Geometry: final body of the model. Coordinates: model frame, mm. Face numbers are marked on the shaded views. A direction names the side the tool comes from. Give positions to 0.01 mm unless a question says otherwise; leave off trailing zeros. Write each loop counter-clockwise with the first axis right and the second up, starting at its lowest first coordinate (ties: lowest second). Pieces come first, ordered by that corner, then holes. Notation, with made-up numbers: (4, 59.25) - (25, 59.25) arc R18 cw to (25, 86.25) - close; hole circle Ø11 at (-19, 79). An arc over 180 degrees is marked (long way). One line per question, with ' | ' between items. Start each with the question number.
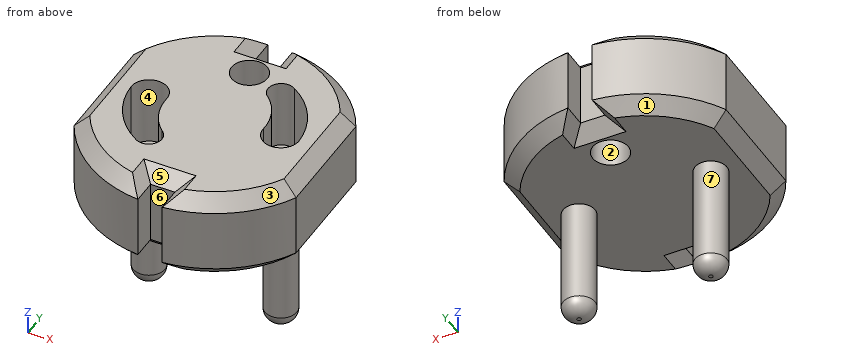
```python
from build123d import *

# Parameters (mm, degrees)
F0_R     = 2.575
F1_DEPTH = 13
F0_R_2   = 2.3
F2_DEPTH = 3
F3_DEPTH = 17
F4_R     = 2
F5_SIZE  = 1.99999
F6_SIZE  = 1.99999


# Not quite as in the source:
# - a fillet or chamfer is up to 0.001 mm smaller than in the source, because OpenCascade refuses the exact size


with BuildPart() as f1:
    # F0 (on Top) → F1 (new body)
    with BuildSketch(Plane.XY):
        with BuildLine():
            Line((1.75, -14.4147285773), (1.75, -17.9147285773))
            ThreePointArc((1.75, -17.9147285773), (10.1062199571, -14.895110546), (16, -8.2462112512))
            Line((16, -8.2462112512), (16, 8.2462112512))
            ThreePointArc((16, 8.2462112512), (10.1062199571, 14.895110546), (1.75, 17.9147285773))
            Line((1.75, 17.9147285773), (1.75, 14.4147285773))
            Line((1.75, 14.4147285773), (-1.75, 14.4147285773))
            Line((-1.75, 14.4147285773), (-1.75, 17.9147285773))
            ThreePointArc((-1.75, 17.9147285773), (-10.1062199571, 14.895110546), (-16, 8.2462112512))
            Line((-16, 8.2462112512), (-16, -8.2462112512))
            ThreePointArc((-16, -8.2462112512), (-10.1062199571, -14.895110546), (-1.75, -17.9147285773))
            Line((-1.75, -17.9147285773), (-1.75, -14.4147285773))
            Line((-1.75, -14.4147285773), (1.75, -14.4147285773))
        make_face()
        with BuildLine():
            ThreePointArc((-12.1, 0), (-9.4098118123, 2.5984353159), (-6.9062568532, -0.1802678246))
            ThreePointArc((-6.9062568532, -0.1802678246), (-6.3236870302, -3.4718300474), (-4.3937995375, -6.2011713107))
            ThreePointArc((-4.3937995375, -6.2011713107), (-3.9419565942, -8.8499140227), (-6.5906993063, -9.301756966))
            ThreePointArc((-6.5906993063, -9.301756966), (-10.5283348632, -5.3515440951), (-12.1, 0))
        make_face(mode=Mode.SUBTRACT)
        with BuildLine():
            ThreePointArc((12.1, 0), (9.4098118123, -2.5984353159), (6.9062568532, 0.1802678246))
            ThreePointArc((6.9062568532, 0.1802678246), (6.3236870302, 3.4718300474), (4.3937995375, 6.2011713107))
            ThreePointArc((4.3937995375, 6.2011713107), (3.9419565942, 8.8499140227), (6.5906993063, 9.301756966))
            ThreePointArc((6.5906993063, 9.301756966), (10.5283348632, 5.3515440951), (12.1, 0))
        make_face(mode=Mode.SUBTRACT)
        with Locations((0, 9.5)):
            Circle(F0_R, mode=Mode.SUBTRACT)
    extrude(amount=F1_DEPTH)

    # F0 (on Top) → F2 (join)
    with BuildSketch(Plane.XY):
        with BuildLine():
            ThreePointArc((-4.3937995375, -6.2011713107), (-6.3236870302, -3.4718300474), (-6.9062568532, -0.1802678246))
            ThreePointArc((-6.9062568532, -0.1802678246), (-9.4098118123, 2.5984353159), (-12.1, 0))
            ThreePointArc((-12.1, 0), (-10.5283348632, -5.3515440951), (-6.5906993063, -9.301756966))
            ThreePointArc((-6.5906993063, -9.301756966), (-3.9419565942, -8.8499140227), (-4.3937995375, -6.2011713107))
        make_face()
        with Locations((-9.5, 0)):
            Circle(F0_R_2, mode=Mode.SUBTRACT)
        with Locations((-9.5, 0)):
            Circle(F0_R_2)
        with BuildLine():
            ThreePointArc((4.3937995375, 6.2011713107), (6.3236870302, 3.4718300474), (6.9062568532, 0.1802678246))
            ThreePointArc((6.9062568532, 0.1802678246), (9.4098118123, -2.5984353159), (12.1, 0))
            ThreePointArc((12.1, 0), (10.5283348632, 5.3515440951), (6.5906993063, 9.301756966))
            ThreePointArc((6.5906993063, 9.301756966), (3.9419565942, 8.8499140227), (4.3937995375, 6.2011713107))
        make_face()
        with Locations((9.5, 0)):
            Circle(F0_R_2, mode=Mode.SUBTRACT)
        with Locations((9.5, 0)):
            Circle(F0_R_2)
    extrude(amount=F2_DEPTH)

    # F0 (on Top) → F3 (join)
    with BuildSketch(Plane.XY):
        with Locations((-9.5, 0)):
            Circle(F0_R_2)
        with Locations((9.5, 0)):
            Circle(F0_R_2)
    extrude(amount=-F3_DEPTH)

    # F4
    f4_edges = [f1.edges().sort_by_distance(p)[0] for p in [
        (-11.8, 0, -17),
        (7.2, 0, -17),
    ]]
    fillet(f4_edges, radius=F4_R)

    # F5 (size 2 in the source; OpenCascade refuses exactly that, so slightly less here)
    f5_edges = [f1.edges().sort_by_distance(p)[0] for p in [
        (10.10622, 14.895111, 13),
        (16, 0, 13),
        (10.10622, -14.895111, 13),
        (1.75, -16.164729, 13),
        (0, -14.414729, 13),
        (-1.75, -16.164729, 13),
        (-10.10622, -14.895111, 13),
        (-16, 0, 13),
        (-10.10622, 14.895111, 13),
        (-1.75, 16.164729, 13),
        (0, 14.414729, 13),
        (1.75, 16.164729, 13),
    ]]
    chamfer(f5_edges, length=F5_SIZE)

    # F6 (size 2 in the source; OpenCascade refuses exactly that, so slightly less here)
    f6_edges = [f1.edges().sort_by_distance(p)[0] for p in [
        (10.10622, 14.895111, 0),
        (16, 0, 0),
        (10.10622, -14.895111, 0),
        (0, 14.414729, 0),
        (1.75, 16.164729, 0),
        (-1.75, 16.164729, 0),
        (-10.10622, 14.895111, 0),
        (-16, 0, 0),
        (-10.10622, -14.895111, 0),
        (-1.75, -16.164729, 0),
        (0, -14.414729, 0),
        (1.75, -16.164729, 0),
    ]]
    chamfer(f6_edges, length=F6_SIZE)


solid = f1.part
```
1) Pull-direction query (Y, two-part tool) for the marked faces 1, 2, 3 and 4; classes: +Y half, -Y half, draft (parallel to the pull), parting line (faces both ways), or undercut.
2) Reachability of the marked faces 5, 6 and 7 from +Z, -Z, +X, -X, +Y, -Y: full face, straight path, thin tool, end or side. Return the list, or none.
3) Line query: L1, parallel to X at y = 9, z = 9; L2, parallel to Y at x = 0, z = 9.75 (3 decimals); L3, parallel to Z at x = -13.5, y = -7. Output: solid intervals per line, ascending.
4) Section A-A, the plane x = 0. Output: boundary loops of the cut face in (y, z) (3 decimals), plus the area to 3 significant figures.
5) First-contact query: pin 1 Ø1.5 at (y, z) = (-9.5, 8.5) entering from -X; pin 2 Ø5 at (y, z) = (0.5, -8.5) entering from +X; pin 3 Ø1 at (y, z) = (-15.5, 4.5) entering from -X. Flat tips, straight axial feed; report the tip coordinate or a pass-through.
6) Section D-D, the plane y = -4.5. Output: boundary loops of the cut face in (x, z), plus the area to 3 significant figures.
7) Section B-B, the plane z = 5.5. Output: boundary loops of the cut face in (x, y) (3 decimals).
8) Section C-C, the plane z = -0.5. Output: boundary loops of the cut face in (x, y), plus the area to 3 significant figures.
Answer key:
1) face 1: +Y half | face 2: undercut | face 3: -Y half | face 4: undercut
2) face 5: +Z, -Y | face 6: +Z, -Z, -Y | face 7: -Z
3) L1: -15.59 to -2.53, 2.53 to 4.06, 7.07 to 15.59 | L2: -14.415 to 6.925, 12.075 to 14.415 | L3: 0 to 13
4) outline: (-14.415, 2) - (-12.415, 0) - (6.925, 0) - (6.925, 13) - (-12.415, 13) - (-14.415, 11) - close; (12.075, 0) - (12.415, 0) - (14.415, 2) - (14.415, 11) - (12.415, 13) - (12.075, 13) - close | area: 300 mm^2
5) pin 1: x = -15.73 | pin 2: x = 11.8 | pin 3: x = -9.95
6) outline: (-16, 2) - (-14, 0) - (14, 0) - (16, 2) - (16, 11) - (14, 13) - (-5.8, 13) - (-5.8, 3) - (-10.98, 3) - (-10.98, 13) - (-14, 13) - (-16, 11) - close | area: 356 mm^2
7) outline: (-16, -8.246) arc R18 ccw to (-1.75, -17.915) - (-1.75, -14.415) - (1.75, -14.415) - (1.75, -17.915) arc R18 ccw to (16, -8.246) - (16, 8.246) arc R18 ccw to (1.75, 17.915) - (1.75, 14.415) - (-1.75, 14.415) - (-1.75, 17.915) arc R18 ccw to (-16, 8.246) - close; hole (-12.1, 0) arc R11.313 ccw to (-6.591, -9.302) arc R1.9 ccw to (-4.394, -6.201) arc R7.654 cw to (-6.906, -0.18) arc R2.6 ccw (long way) to start; hole circle Ø5.15 at (0, 9.5); hole (4.394, 6.201) arc R7.654 cw to (6.906, 0.18) arc R2.6 ccw (long way) to (12.1, 0) arc R11.313 ccw to (6.591, 9.302) arc R1.9 ccw to start
8) outline: circle Ø4.6 at (-9.5, 0); circle Ø4.6 at (9.5, 0) | area: 33.2 mm^2
